The model under review builds one solid part; all positions refer to its coordinate system, in mm. A direction names the side the tool comes from. Round coordinates to 2 decimals unless told otherwise and drop trailing zeros. Write each loop counter-clockwise with the first axis right and the second up, starting at its lowest first coordinate (ties: lowest second). Pieces come first, ordered by that corner, then holes. Notation, with made-up numbers: M 32.25,8.25 L 84.25,8.25 A23 ccw 84.25,40.25 Z; hole C -14,30 d9. An arc over 180 degrees is marked long. Write item = value, one per line. Start each with the question number.
Item 1: Take a section at B-B, the plane z = 856.5. Give the boundary of the cut face in (x, y), plus the area to 4 significant figures.
Item 2: Take a section at A-A, the plane y = 8640.5. Give the boundary of the cut face in (x, z).
Item 3: The part is to be moulded in two halves that separate along Z. For faces 1 (the cylindrical face through (7430.31, 8333.998, 1079.227)), 2 (the cylindrical face through (7430.31, 8773.998, 1079.227)), 3 (the flat face through (6645, 8213.208, 740)), 4 (the flat face through (6645, 8796, 1500)), say which applies: +Z half, -Z half, draft (parallel to the pull), parting line (faces both ways), or undercut.
Item 4: For pin 1 Ø25 at (x, z) = (7428.5, 1337.5) entering from +Y, flat-tipped, find the tip position at first contact; note if it passes through.
Item 5: Tool access review of faces 5 (the cylindrical face through (7430.31, 9213.998, 939.227)), 6 (the flat face through (7455.66, 9013, 945)): name each direction out of +Z, -Z, +X, -X, +Y, -Y from which nothing blocks a thin tool from reaching the whole face with its end or side.
Item 6: To check wall thickness, follow line 1 along X through (y, z) = (8632.5, 861). State the ranges of the line that lie inside material, in increasing order.
from build123d import *

# Parameters (mm, degrees)
SKETCH1_W           = 1500
SKETCH1_H           = 1150
BOSS_EXTRUDE1_DEPTH = 1500
SKETCH2_R           = 20
SKETCH2_W           = 241.410698637
SKETCH2_H           = 880
BOSS_EXTRUDE2_DEPTH = 50


with BuildPart() as part:
    # Sketch1 → Boss-Extrude1 (new body)
    with BuildSketch(Plane.XY):
        with Locations((6655.660377358, 8788.20754717)):
            Rectangle(SKETCH1_W, SKETCH1_H)
    extrude(amount=BOSS_EXTRUDE1_DEPTH)

    # Sketch2 → Boss-Extrude2 (add)
    with BuildSketch(Plane(origin=(7405.660377359, 0, 0), x_dir=(0, 0, -1), z_dir=(1, 0, 0))):
        with Locations(Location((-1085.234472632, 8353.074404115, 0), (0, 0, 270))):
            Circle(SKETCH2_R)
        with Locations(Location((-945.234472632, 8353.074404115, 0), (0, 0, 270))):
            Circle(SKETCH2_R)
        with Locations(Location((-945.234472632, 8573.074404115, 0), (0, 0, 270))):
            Circle(SKETCH2_R)
        with Locations(Location((-945.234472632, 8793.074404115, 0), (0, 0, 270))):
            Circle(SKETCH2_R)
        with Locations(Location((-945.234472632, 9013.074404115, 0), (0, 0, 270))):
            Circle(SKETCH2_R)
        with Locations(Location((-945.234472632, 9233.074404115, 0), (0, 0, 270))):
            Circle(SKETCH2_R)
        with Locations(Location((-1085.234472632, 8573.074404115, 0), (0, 0, 270))):
            Circle(SKETCH2_R)
        with Locations(Location((-1085.234472632, 8793.074404115, 0), (0, 0, 270))):
            Circle(SKETCH2_R)
        with Locations(Location((-1085.234472632, 9013.074404115, 0), (0, 0, 270))):
            Circle(SKETCH2_R)
        with Locations(Location((-1085.234472632, 9233.074404115, 0), (0, 0, 270))):
            Circle(SKETCH2_R)
        with Locations((-1293.028757662, 8793.074404115)):
            Rectangle(SKETCH2_W, SKETCH2_H)
    extrude(amount=BOSS_EXTRUDE2_DEPTH)


solid = part.part
Response values:
q1.outline = M 5905.66,8213.21 L 7405.66,8213.21 L 7405.66,9363.21 L 5905.66,9363.21 Z
q1.area = 1,725,000 mm2
q2.outline = M 5905.66,0 L 7405.66,0 L 7405.66,1172.32 L 7455.66,1172.32 L 7455.66,1413.73 L 7405.66,1413.73 L 7405.66,1500 L 5905.66,1500 Z
q3.face_1 = undercut
q3.face_2 = undercut
q3.face_3 = draft
q3.face_4 = +Z half
q4.pin_1 = 9233.07
q5.face_5 = +X
q5.face_6 = +Z, -Z, +X, +Y, -Y
q6.line_1 = 5905.66 to 7405.66
